Verification items for the finished model (mm, model axes). A direction names the side the tool comes from. Give positions to 0.01 mm unless a question says otherwise; leave off trailing zeros. Write each loop counter-clockwise with the first axis right and the second up, starting at its lowest first coordinate (ties: lowest second). Pieces come first, ordered by that corner, then holes. Notation, with made-up numbers: M 65.5,-38.75 L 99.5,-38.75 A20 ccw 99.5,-27.75 Z; hole C -37,32 d6. An arc over 180 degrees is marked long. Write item = value, one per line.
Solid Edge part; units mm, degrees
sketch "Sketch1" plane through (0, 0, 0) normal (0, 0, 1) x (1, 0, 0)
  arc A0 (-2.3476, -7.7448) -> (-3.4125, -6.3093) centre (-1.9125, -6.3093) cw
  arc A1 (-4.4168, -3.8295) -> (-3.4125, -6.3093) centre (-6.976, -6.3093) cw
  arc A2 (-4.4168, -3.8295) -> (4.4168, -3.8295) centre (0, 0.45) cw
  arc A3 (4.4168, -3.8295) -> (3.4125, -6.3093) centre (6.976, -6.3093) ccw
  arc A4 (2.3476, -7.7448) -> (3.4125, -6.3093) centre (1.9125, -6.3093) ccw
  arc A5 (2.3476, -7.7448) -> (0.4125, -8.0822) centre (0, 0) cw
  line L0 (0.4125, -8.0822) -> (0.4125, -4.7822)
  arc A6 (-0.4125, -4.7822) -> (0.4125, -4.7822) centre (0, 0) cw
  line L1 (-0.4125, -8.0822) -> (-0.4125, -4.7822)
  arc A7 (-0.4125, -8.0822) -> (-2.3476, -7.7448) centre (0, 0) cw
extrude "Protrusion1" add sketch "Sketch1" along normal blind 1
sketch "Sketch2" plane through (0, 0, 0) normal (0, 0, 1) x (1, 0, 0)
  circle A0 centre (-1.9125, -6.3093) radius 0.75
extrude "Cutout1" cut sketch "Sketch2" along normal through all
sketch "Sketch3" plane through (0, 0, 0) normal (0, 0, 1) x (1, 0, 0)
  circle A0 centre (1.9125, -6.3093) radius 0.75
extrude "Cutout2" cut sketch "Sketch3" along normal through all
properties material "Stahl"
1) Cross-section at C-C on x = 0.75. Record the boundary of the cut face in (y, z), plus the area to 3 significant figures.
From the geometry:
outline = M -8.06,0 L -4.74,0 L -4.74,1 L -8.06,1 Z; M 4.74,0 L 6.55,0 L 6.55,1 L 4.74,1 Z
area = 5.13 mm^2
2) Tool access check on faces 1 (the flat face through (0.413, -6.5, 0.5)), 2 (the cylindrical face through (3.125, -7.192, 0.493)). Record the directions out of +Z, -Z, +X, -X, +Y, -Y that give a thin tool (end or side, any length) a straight path to the whole face; none if there is none.
From the geometry:
face_1 = +Z, -Z, -Y
face_2 = +Z, -Z, +X, -Y
3) Cross-section at A-A on y = -0.25. Record the boundary of the cut face in (x, z), plus the area to 3 significant figures.
From the geometry:
outline = M -6.11,0 L -4.79,0 L -4.79,1 L -6.11,1 Z; M 4.79,0 L 6.11,0 L 6.11,1 L 4.79,1 Z
area = 2.63 mm^2
4) Material ranges on probe 1 along Y at (x, z) = (0, 0.4); probe 2 along Y at (x, z) = (2.25, 0.8); probe 3 along Y at (x, z) = (-2, 0.55), recorded low to high. Write a range as from..to.
From the geometry:
probe_1 = 4.8..6.6
probe_2 = -7.77..-6.98, -5.64..-4.24, 4.24..6.17
probe_3 = -7.84..-7.05, -5.56..-4.36, 4.36..6.27
5) Draft check along Y on faces 3 (the flat face through (-0.413, -6.5, 0.5)), 4 (the cylindrical face through (1.75, -5.577, 0.493)), 5 (the cylindrical face through (1.4, -7.97, 0.49)). Enter one of: +Y half, -Y half, draft (parallel to the pull), parting line (faces both ways), or undercut.
From the geometry:
face_3 = draft
face_4 = undercut
face_5 = -Y half
6) Depth check by flat-ended pin: P1, Ø0.5, axis at y = -6.5, z = 0.5, coming from the +X side; P2, Ø1.7, axis at x = -1.91, y = -6.31, coming from the +Z side. Enter the tip coordinate at first touch or a pass-through.
From the geometry:
P1 = 3.41
P2 = 1
7) Cross-section at B-B on x = 2. Record the boundary of the cut face in (y, z), plus the area to 3 significant figures.
From the geometry:
outline = M -7.84,0 L -7.05,0 L -7.05,1 L -7.84,1 Z; M -5.56,0 L -4.36,0 L -4.36,1 L -5.56,1 Z; M 4.36,0 L 6.27,0 L 6.27,1 L 4.36,1 Z
area = 3.89 mm^2
8) Cross-section at D-D on z = 0.75. Record the boundary of the cut face in (x, y).
From the geometry:
outline = M -4.42,-3.83 A3.56 cw -3.41,-6.31 A1.5 ccw -2.35,-7.74 A8.09 ccw -0.41,-8.08 L -0.41,-4.78 A4.8 cw long 0.41,-4.78 L 0.41,-8.08 A8.09 ccw 2.35,-7.74 A1.5 ccw 3.41,-6.31 A3.56 cw 4.42,-3.83 A6.15 ccw long Z; hole C -1.91,-6.31 d1.5; hole C 1.91,-6.31 d1.5
